Check sheet for the modelled part. Datum: model origin and axes. Units: mm. Give positions to 0.01 mm unless a question says otherwise; leave off trailing zeros. Order: outer loops, then holes, each group sorted by start corner. A loop starts at its lowest first (then second) coordinate and runs counter-clockwise, first axis right, second up. Notation, with made-up numbers: (43, 57.25) -> (65, 57.25) arc R22 cw to (65, 81.25) -> close; hole circle Ø6 at (-27.75, 82.25). An arc over 180 degrees is marked (long way). Write each question's results on one line, items separated by ' | '.
from build123d import *

# Parameters (mm, degrees)
SKETCH1_R           = 0.7
BOSS_EXTRUDE2_DEPTH = 5


with BuildPart() as part:
    # Sketch1 → Boss-Extrude2 (new body)
    with BuildSketch(Plane.XY):
        with BuildLine():
            Line((3.25, -6.019172648), (-3.25, -6.019172648))
            ThreePointArc((-3.25, -6.019172648), (-6.268760929, -4.768760929), (-7.519172648, -1.75))
            Line((-7.519172648, -1.75), (-7.519172648, 3.25))
            Line((-7.519172648, 3.25), (7.519172648, 3.25))
            Line((7.519172648, 3.25), (7.519172648, -1.75))
            ThreePointArc((7.519172648, -1.75), (6.268760929, -4.768760929), (3.25, -6.019172648))
        make_face()
        with Locations((-3.25, -1.75)):
            Circle(SKETCH1_R, mode=Mode.SUBTRACT)
        with Locations((3.25, -1.75)):
            Circle(SKETCH1_R, mode=Mode.SUBTRACT)
    extrude(amount=BOSS_EXTRUDE2_DEPTH)


solid = part.part
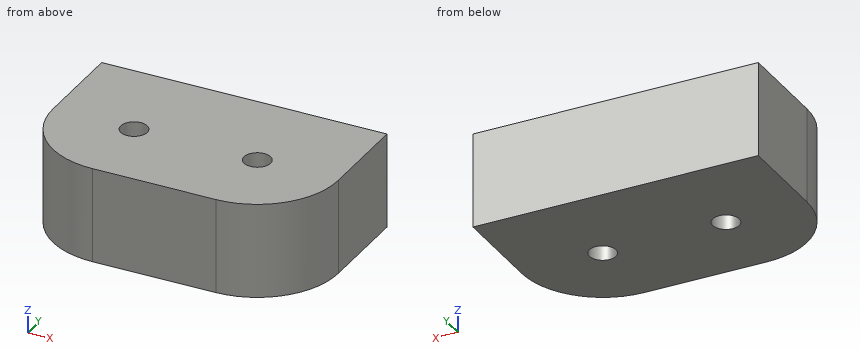
1. Section check A-A on z = 4.3. Record the cut outline in (x, y).
Verdict:
outline: (-7.52, -1.75) arc R4.27 ccw to (-3.25, -6.02) -> (3.25, -6.02) arc R4.27 ccw to (7.52, -1.75) -> (7.52, 3.25) -> (-7.52, 3.25) -> close; hole circle Ø1.4 at (-3.25, -1.75); hole circle Ø1.4 at (3.25, -1.75)
2. Section check B-B on x = -2.75. Record the cut outline in (y, z), then the cut area to 3 significant figures.
Verdict:
outline: (-6.02, 0) -> (-2.24, 0) -> (-2.24, 5) -> (-6.02, 5) -> close; (-1.26, 0) -> (3.25, 0) -> (3.25, 5) -> (-1.26, 5) -> close | area: 41.4 mm^2
3. Gauge pin test, flat end, axial feed: pin 1 Ø1 at (y, z) = (-4.5, 3.5) entering from -X. Record the tip position at first contact, or that the pin passes through.
Verdict:
pin 1: stops at x = -6.88
4. Section check C-C on y = -5. Record the cut outline in (x, z).
Verdict:
outline: (-6.02, 0) -> (6.02, 0) -> (6.02, 5) -> (-6.02, 5) -> close
5. Material ranges on probe 1 along Y at (x, z) = (-3.25, 2.85); probe 2 along Y at (x, z) = (-5.5, 2.85); probe 3 along X at (y, z) = (-2.5, 2.2), recorded low to high. Write a range as from..to.
Verdict:
probe 1: y = -6.02..-2.45, -1.05..3.25 | probe 2: y = -5.38..3.25 | probe 3: x = -7.45..7.45
6. Section check D-D on x = 4.75. Record the cut outline in (y, z), then the cut area to 3 significant figures.
Verdict:
outline: (-5.75, 0) -> (3.25, 0) -> (3.25, 5) -> (-5.75, 5) -> close | area: 45.0 mm^2
